Verification items for the finished model (mm, model axes). Give positions to 0.01 mm unless a question says otherwise; leave off trailing zeros. Write each loop counter-clockwise with the first axis right and the second up, starting at its lowest first coordinate (ties: lowest second). Pieces come first, ordered by that corner, then holes. Notation, with made-up numbers: M -33,-35 L -22,-35 A14 cw -22,-11 Z; hole C -15.75,57 d3. An arc over 180 degrees is marked long. Write item = value, one per line.
from build123d import *

# Parameters (mm, degrees)
SKIZZE1_R                       = 70
SKIZZE1_R_2                     = 15
AUFSATZ_LINEAR_AUSTRAGEN1_DEPTH = 8
SKIZZE2_R                       = 1.7
SCHNITT_LINEAR_AUSTRAGEN1_DEPTH = 8
SKIZZE3_R                       = 3
SCHNITT_LINEAR_AUSTRAGEN2_DEPTH = 3
SCHNITT_LINEAR_AUSTRAGEN3_DEPTH = 8


with BuildPart() as part:
    # Skizze1 → Aufsatz-Linear austragen1 (new body)
    with BuildSketch(Plane(origin=(0, 0, 0), x_dir=(0, 1, 0), z_dir=(0, 0, 1))):
        with Locations(Location((0, 0, 0), (0, 0, 270))):
            Circle(SKIZZE1_R)
        with Locations(Location((0, 0, 0), (0, 0, 270))):
            Circle(SKIZZE1_R_2, mode=Mode.SUBTRACT)
    extrude(amount=AUFSATZ_LINEAR_AUSTRAGEN1_DEPTH)

    # Skizze2 → Schnitt-Linear austragen1 (cut)
    with BuildSketch(Plane.XY.offset(8)):
        with Locations((0, 65)):
            Circle(SKIZZE2_R)
        with Locations((64.837196687, 0.18986002)):
            Circle(SKIZZE2_R)
        with Locations((0, -65)):
            Circle(SKIZZE2_R)
        with Locations((-65, 0)):
            Circle(SKIZZE2_R)
    extrude(amount=-SCHNITT_LINEAR_AUSTRAGEN1_DEPTH, mode=Mode.SUBTRACT)

    # Skizze3 → Schnitt-Linear austragen2 (cut)
    with BuildSketch(Plane.XY.offset(8)):
        with Locations((0, 65)):
            Circle(SKIZZE3_R)
        with Locations((64.837196687, 0.18986002)):
            Circle(SKIZZE3_R)
        with Locations((0, -65)):
            Circle(SKIZZE3_R)
        with Locations((-65, 0)):
            Circle(SKIZZE3_R)
    extrude(amount=-SCHNITT_LINEAR_AUSTRAGEN2_DEPTH, mode=Mode.SUBTRACT)

    # Skizze4 → Schnitt-Linear austragen3 (cut)
    with BuildSketch(Plane.XY.offset(8)):
        Polygon((66.550324449, -89.690139622), (8.405353871, -34.743234372), (32.444624917, -9.304809744), (90.589595495, -64.251714994), align=None)
    extrude(amount=-SCHNITT_LINEAR_AUSTRAGEN3_DEPTH, mode=Mode.SUBTRACT)


solid = part.part
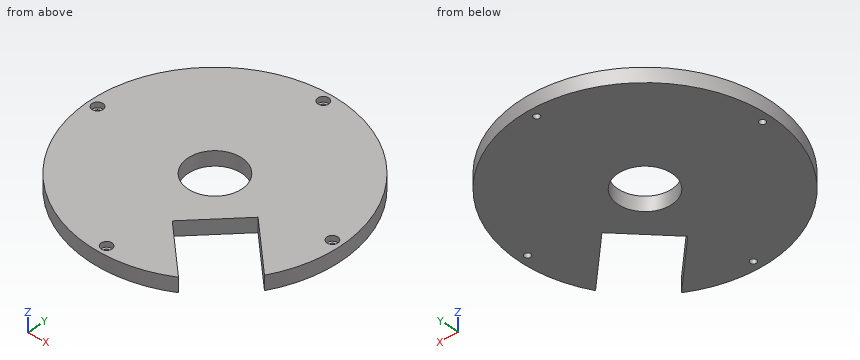
1) Depth check by flat-ended pin: P1, Ø5.5, axis at x = 0, y = 65, coming from the +Z side; P2, Ø2, axis at y = 43.5, z = 6, coming from the +X side. Enter the tip coordinate at first touch or a pass-through.
From the geometry:
P1 = 5
P2 = 55.62
2) Cross-section at A-A on x = 0. Record the boundary of the cut face in (y, z), plus the area to 3 significant figures.
From the geometry:
outline = M -70,0 L -66.7,0 L -66.7,5 L -68,5 L -68,8 L -70,8 Z; M -63.3,0 L -15,0 L -15,8 L -62,8 L -62,5 L -63.3,5 Z; M 15,0 L 63.3,0 L 63.3,5 L 62,5 L 62,8 L 15,8 Z; M 66.7,0 L 70,0 L 70,8 L 68,8 L 68,5 L 66.7,5 Z
area = 810 mm^2
3) Material ranges on probe 1 along Y at (x, z) = (11, 3); probe 2 along X at (y, z) = (2, 7.25); probe 3 along X at (y, z) = (1.5, 1), recorded low to high. Write a range as from..to.
From the geometry:
probe_1 = -69.13..-37.2, -32..-10.2, 10.2..69.13
probe_2 = -69.97..-67.24, -62.76..-14.87, 14.87..62.44, 67.23..69.97
probe_3 = -69.98..-65.8, -64.2..-14.92, 14.92..63.75, 65.92..69.98
4) Cross-section at B-B on y = 65. Record the boundary of the cut face in (x, z).
From the geometry:
outline = M -25.98,0 L -1.7,0 L -1.7,5 L -3,5 L -3,8 L -25.98,8 Z; M 1.7,0 L 25.98,0 L 25.98,8 L 3,8 L 3,5 L 1.7,5 Z
5) Cross-section at C-C on z = 6.75. Record the boundary of the cut face in (x, y).
From the geometry:
outline = M 8.41,-34.74 L 32.44,-9.3 L 60.27,-35.6 A70 ccw long 35.49,-60.34 Z; hole C -65,0 d6; hole C 0,0 d30; hole C 0,-65 d6; hole C 0,65 d6; hole C 64.84,0.19 d6
